Could you check a few things on this model? Use its own coordinates, in mm. A direction names the side the tool comes from. Coordinates: 2 decimals unless noted, no trailing zeros. Order: outer loops, then holes, each group sorted by start corner. A loop starts at its lowest first (then second) coordinate and runs counter-clockwise, first axis right, second up. Notation, with made-up numbers: M 55.25,16 L 78.25,16 A29 ccw 78.25,55 Z; hole C -2,-14 d3. An arc over 180 degrees is marked long. One line per question, with ' | ' between items. Start each with the question number.
from build123d import *

# Parameters (mm, degrees)
SKETCH1_W            = 2
SKETCH1_H            = 32.4
SKETCH1_W_2          = 5
SKETCH1_H_2          = 3
SKETCH1_W_3          = 3
SKETCH1_W_4          = 8
BOSS_EXTRUDE1_DEPTH  = 3
BOSS_EXTRUDE2_DEPTH  = 27
SKETCH1_4_W          = 5
SKETCH1_4_H          = 3
SKETCH1_4_W_2        = 3
BOSS_EXTRUDE3_DEPTH  = 16
SKETCH1_5_W          = 8
SKETCH1_5_H          = 3
BOSS_EXTRUDE4_DEPTH  = 11
SKETCH1_6_W          = 2
SKETCH1_6_H          = 32.4
BOSS_EXTRUDE5_DEPTH  = 26
BOSS_EXTRUDE6_DEPTH  = 27
SKETCH3_W            = 31.6
SKETCH3_H            = 48.4
BOSS_EXTRUDE7_DEPTH  = 3
BOSS_EXTRUDE8_DEPTH  = 3
BOSS_EXTRUDE9_DEPTH  = 3
SKETCH6_R            = 1.5
CUT_EXTRUDE1_DEPTH   = 10
SKETCH7_W            = 2
SKETCH7_H            = 9.25
BOSS_EXTRUDE10_DEPTH = 4


with BuildPart() as part:
    # Sketch1 → Boss-Extrude1 (new body)
    with BuildSketch(Plane.XY):
        Polygon((3, 0), (0, 0), (-3, 0), (-22.6, 0), (-22.6, 27), (-25.6, 27), (-25.6, -3), (0, -3), (5.5, -3), (5.5, 0), align=None)
        Polygon((0, 62.4), (0, 47.2), (0, 44.2), (0, 41.2), (0, 3), (0, 0), (-3, 0), (-3, 27), (-4.55, 27), (-4.55, 59.4), (-21.05, 59.4), (-21.05, 27), (-22.6, 27), (-25.6, 27), (-25.6, 59.4), (-25.6, 62.4), (-4.55, 62.4), align=None)
        with Locations((-20.05, 43.2)):
            Rectangle(SKETCH1_W, SKETCH1_H)
        Polygon((-22.6, 0), (-3, 0), (-3, 27), (-4.55, 27), (-6.55, 27), (-6.55, 59.4), (-19.05, 59.4), (-19.05, 27), (-21.05, 27), (-22.6, 27), align=None)
        with Locations((2.5, 42.7)):
            Rectangle(SKETCH1_W_2, SKETCH1_H_2)
        Polygon((0, 47.2), (0, 44.2), (5, 44.2), (14, 44.2), (19, 44.2), (19, 41.2), (19, 3), (19, 0), (22, 0), (22, 44.2), (22, 47.2), align=None)
        with Locations((16.5, 42.7)):
            Rectangle(SKETCH1_W_2, SKETCH1_H_2)
        Polygon((3, 3), (3, 0), (5.5, 0), (13.5, 0), (16, 0), (16, 3), (19, 3), (19, 41.2), (14, 41.2), (14, 44.2), (5, 44.2), (5, 41.2), (0, 41.2), (0, 3), align=None)
        with Locations((17.5, 1.5)):
            Rectangle(SKETCH1_W_3, SKETCH1_H_2)
        Polygon((16, 0), (13.5, 0), (13.5, -3), (22, -3), (22, 0), (19, 0), align=None)
        with Locations((1.5, 1.5)):
            Rectangle(SKETCH1_W_3, SKETCH1_H_2)
        with Locations((9.5, -1.5)):
            Rectangle(SKETCH1_W_4, SKETCH1_H_2)
        with Locations((-5.55, 43.2)):
            Rectangle(SKETCH1_W, SKETCH1_H)
    extrude(amount=BOSS_EXTRUDE1_DEPTH)

    # Sketch1<3> → Boss-Extrude2 (add)
    with BuildSketch(Plane.XY):
        Polygon((0, 62.4), (0, 47.2), (0, 44.2), (0, 41.2), (0, 3), (0, 0), (-3, 0), (-3, 27), (-4.55, 27), (-4.55, 59.4), (-21.05, 59.4), (-21.05, 27), (-22.6, 27), (-25.6, 27), (-25.6, 59.4), (-25.6, 62.4), (-4.55, 62.4), align=None)
        Polygon((3, 0), (0, 0), (-3, 0), (-22.6, 0), (-22.6, 27), (-25.6, 27), (-25.6, -3), (0, -3), (5.5, -3), (5.5, 0), align=None)
        Polygon((16, 0), (13.5, 0), (13.5, -3), (22, -3), (22, 0), (19, 0), align=None)
        Polygon((0, 47.2), (0, 44.2), (5, 44.2), (14, 44.2), (19, 44.2), (19, 41.2), (19, 3), (19, 0), (22, 0), (22, 44.2), (22, 47.2), align=None)
    extrude(amount=BOSS_EXTRUDE2_DEPTH)

    # Sketch1<4> → Boss-Extrude3 (add)
    with BuildSketch(Plane.XY):
        with Locations((2.5, 42.7)):
            Rectangle(SKETCH1_4_W, SKETCH1_4_H)
        with Locations((16.5, 42.7)):
            Rectangle(SKETCH1_4_W, SKETCH1_4_H)
        with Locations((17.5, 1.5)):
            Rectangle(SKETCH1_4_W_2, SKETCH1_4_H)
        with Locations((1.5, 1.5)):
            Rectangle(SKETCH1_4_W_2, SKETCH1_4_H)
    extrude(amount=BOSS_EXTRUDE3_DEPTH)

    # Sketch1<5> → Boss-Extrude4 (add)
    with BuildSketch(Plane.XY):
        with Locations((9.5, -1.5)):
            Rectangle(SKETCH1_5_W, SKETCH1_5_H)
    extrude(amount=BOSS_EXTRUDE4_DEPTH)

    # Sketch1<6> → Boss-Extrude5 (add)
    with BuildSketch(Plane.XY):
        with Locations((-5.55, 43.2)):
            Rectangle(SKETCH1_6_W, SKETCH1_6_H)
        with Locations((-20.05, 43.2)):
            Rectangle(SKETCH1_6_W, SKETCH1_6_H)
    extrude(amount=BOSS_EXTRUDE5_DEPTH)

    # Sketch2 → Boss-Extrude6 (add)
    with BuildSketch(Plane(origin=(0, 0, 0), x_dir=(-1, 0, 0), z_dir=(0, 0, -1))):
        Polygon((25.6, 0), (25.6, -3), (60.2, -3), (60.2, 58.4), (25.6, 58.4), (25.6, 55.4), (57.2, 55.4), (57.2, 48.4), (57.2, 0), align=None)
    extrude(amount=-BOSS_EXTRUDE6_DEPTH)

    # Sketch3 → Boss-Extrude7 (add)
    with BuildSketch(Plane.XY.offset(27)):
        with Locations((-41.4, 24.2)):
            Rectangle(SKETCH3_W, SKETCH3_H)
    extrude(amount=-BOSS_EXTRUDE7_DEPTH)

    # Sketch4 → Boss-Extrude8 (add)
    with BuildSketch(Plane(origin=(0, -3, 0), x_dir=(-1, 0, 0), z_dir=(0, -1, 0))):
        Polygon((22.6, -42), (22.6, -27), (7.6, -27), align=None)
        Polygon((53.32802139, -27), (22.6, -27), (22.6, -42), (60.2, -42), (60.2, -32.991669089), (54.2, -32.991669089), (54.2, -40.3), (35.4, -40.3), (35.4, -28.7), (53.32802139, -28.7), align=None)
        Polygon((60.2, -27), (53.32802139, -27), (53.32802139, -28.7), (54.2, -28.7), (54.2, -32.991669089), (60.2, -32.991669089), align=None)
    extrude(amount=-BOSS_EXTRUDE8_DEPTH)

    # Sketch5 → Boss-Extrude9 (add)
    with BuildSketch(Plane.ZY.offset(60.2)):
        Polygon((27, 0), (42, 0), (27, 15), align=None)
    extrude(amount=-BOSS_EXTRUDE9_DEPTH)

    # Sketch6 → Cut-Extrude1 (cut)
    with BuildSketch(Plane(origin=(0, 0, 24), x_dir=(-1, 0, 0), z_dir=(0, 0, -1))):
        with Locations((30.1, 41.9)):
            Circle(SKETCH6_R)
        with Locations((30.1, 13.5)):
            Circle(SKETCH6_R)
        with Locations((52.7, 27.7)):
            Circle(SKETCH6_R)
    extrude(amount=-CUT_EXTRUDE1_DEPTH, mode=Mode.SUBTRACT)

    # Sketch7 → Boss-Extrude10 (add)
    with BuildSketch(Plane.XY.offset(27)):
        Polygon((-50.15, 38.95), (-50.15, 27.7), (-48.15, 27.7), (-48.15, 36.95), (-41.4, 36.95), (-34.65, 36.95), (-34.65, 27.7), (-32.65, 27.7), (-32.65, 36.95), (-32.65, 38.95), (-48.15, 38.95), align=None)
        Polygon((-48.15, 27.7), (-50.15, 27.7), (-50.15, 18.45), (-50.15, 16.45), (-32.65, 16.45), (-32.65, 18.45), (-34.65, 18.45), (-41.4, 18.45), (-48.15, 18.45), align=None)
        with Locations((-33.65, 23.075)):
            Rectangle(SKETCH7_W, SKETCH7_H)
    extrude(amount=BOSS_EXTRUDE10_DEPTH)


solid = part.part
(1) We'd pull the mould along Y, two halves only. Please class faces 1 (the flat face through (-3, 13, 15)), 2 (the flat face through (0, 30, 0)), 3 (the flat face through (-43, 58.4, 13)): +Y half, -Y half, draft (parallel to the pull), parting line (faces both ways), or undercut.
(2) On a 3-axis mill with a long thin cutter (end or side, diameter ignored), from which of +Z, -Z, +X, -X, +Y, -Y can I reach the whole of each face in a straight line? I mean faces 4 (the flat face through (-57.2, 4, 31)), 5 (the flat face through (22, 22, 13)), 6 (the flat face through (-54.2, -2, 34)), 7 (the flat face through (-42, 48.4, 26)), 8 (the flat face through (-41, 28, 27)). Say none if no direction works.
(3) For P1, Ø19.5, axis at x = -37, z = 31.5, coming from the +Y side; P2, Ø12, axis at y = 9, z = 37, coming from the +X side; P3, Ø12, axis at y = 57, z = 18, coming from the +X side, each with a flat end and sliding along its axis, tell me the tip position at first contact or that it passes through.
(4) Imagine slicing it at D-D, the plane z = 19. Write out the boundary of the cut face in (x, y).
(5) Imagine slicing it at A-A, the plane z = 34. Write out the boundary of the cut face in (x, y).
(6) If I drill on line 1 along Y through (x, z) = (-30, 25); line 2 along X through (y, z) = (20.5, 24.5); line 3 along X through (y, z) = (43, 18), over which ranges is the centre line in solid material (lowest first)? Write a range as from..to.
(7) Imagine slicing it at C-C, the plane y = 23. Write out the boundary of the cut face in (x, z).
(8) Imagine slicing it at B-B, the plane x = -52.7. Write out the boundary of the cut face in (y, z).
Answers:
1) face 1: undercut | face 2: draft | face 3: +Y half
2) face 4: +Z, +X, +Y | face 5: +Z, -Z, +X, +Y, -Y | face 6: +Y, -Y | face 7: +Z, -Z | face 8: +Z
3) P1: y = 58.4 | P2: x = -57.2 | P3: x = 0
4) outline: M -60.2,-3 L 5.5,-3 L 5.5,0 L 0,0 L 0,44.2 L 19,44.2 L 19,0 L 13.5,0 L 13.5,-3 L 22,-3 L 22,47.2 L 0,47.2 L 0,62.4 L -25.6,62.4 L -25.6,58.4 L -60.2,58.4 Z; hole M -57.2,0 L -25.6,0 L -25.6,55.4 L -57.2,55.4 Z; hole M -22.6,0 L -3,0 L -3,27 L -6.55,27 L -6.55,59.4 L -19.05,59.4 L -19.05,27 L -22.6,27 Z
5) outline: M -60.2,-3 L -54.2,-3 L -54.2,0 L -57.2,0 L -57.2,8 L -60.2,8 Z; M -35.4,-3 L -14.6,-3 L -14.6,0 L -35.4,0 Z
6) line 1: -3..12, 15..40.4, 43.4..48.4, 55.4..58.4 | line 2: -60.2..-22.6, -3..0, 19..22 | line 3: -60.2..-57.2, -25.6..-19.05, -6.55..0, 19..22
7) outline: M -60.2,0 L -57.2,0 L -57.2,24 L -25.6,24 L -25.6,0 L 22,0 L 22,27 L 19,27 L 19,3 L 0,3 L 0,27 L -3,27 L -3,3 L -22.6,3 L -22.6,27 L -32.65,27 L -32.65,31 L -34.65,31 L -34.65,27 L -48.15,27 L -48.15,31 L -50.15,31 L -50.15,27 L -60.2,27 Z
8) outline: M -3,0 L 0,0 L 0,24 L 26.2,24 L 26.2,27 L 0,27 L 0,28.7 L -3,28.7 Z; M -3,40.3 L 0,40.3 L 0,42 L -3,42 Z; M 29.2,24 L 48.4,24 L 48.4,27 L 29.2,27 Z; M 55.4,0 L 58.4,0 L 58.4,27 L 55.4,27 Z
